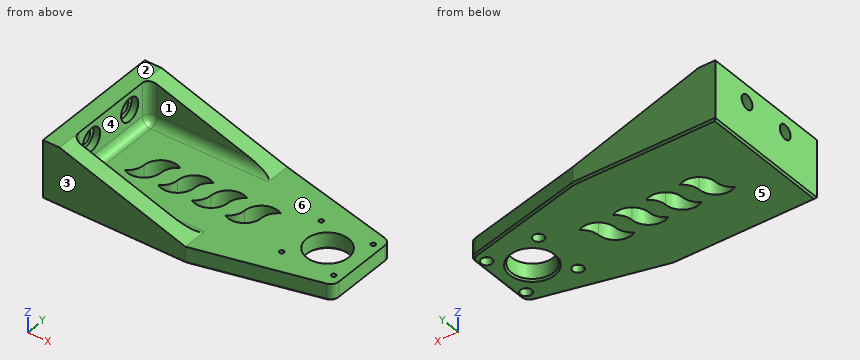
```python
from build123d import *

# Parameters (mm, degrees)
SKETCH1_W           = 160
SKETCH1_H           = 80
BOSS_EXTRUDE1_DEPTH = 10
SKETCH2_R           = 1.325
SKETCH2_R_2         = 12.5
CUT_EXTRUDE1_DEPTH  = 3
CUT_EXTRUDE2_REACH  = 9
SKETCH4_R           = 1.325
SKETCH4_R_2         = 12.5
SKETCH7_W           = 10
SKETCH7_H           = 80
BOSS_EXTRUDE3_DEPTH = 25
BOSS_EXTRUDE4_DEPTH = 10
BOSS_EXTRUDE5_DEPTH = 10
CUT_EXTRUDE3_REACH  = 12
CUT_EXTRUDE4_DEPTH  = 10
FILLET1_R           = 5
SKETCH12_R          = 3.25
CUT_EXTRUDE5_DEPTH  = 4.5
CUT_EXTRUDE6_REACH  = 12
SKETCH13_R          = 4.25
SKETCH14_R          = 6.75
CUT_EXTRUDE7_DEPTH  = 4
FILLET2_R           = 5
CHAMFER2_SIZE       = 1


with BuildPart() as part:
    # Sketch1 → Boss-Extrude1 (new body)
    with BuildSketch(Plane.XY):
        Rectangle(SKETCH1_W, SKETCH1_H)
    extrude(amount=BOSS_EXTRUDE1_DEPTH)

    # Sketch2 → Cut-Extrude1 (cut)
    with BuildSketch(Plane.XY.offset(10)):
        with Locations((44, 15.5)):
            Circle(SKETCH2_R)
        with Locations((75, 15.5)):
            Circle(SKETCH2_R)
        with Locations((44, -15.5)):
            Circle(SKETCH2_R)
        with Locations((75, -15.5)):
            Circle(SKETCH2_R)
        with Locations((59.5, 0)):
            Circle(SKETCH2_R_2)
    extrude(amount=-CUT_EXTRUDE1_DEPTH, mode=Mode.SUBTRACT)

    # Sketch4 → Cut-Extrude2 (cut, up to next)
    with BuildSketch(Plane.XY.offset(7), mode=Mode.PRIVATE) as cut_extrude2_sk1:
        with Locations((75, -15.5)):
            Circle(SKETCH4_R)
    cut_extrude2_tool1 = extrude(cut_extrude2_sk1.sketch, amount=-CUT_EXTRUDE2_REACH, mode=Mode.PRIVATE) & part.part
    add(cut_extrude2_tool1.solids().sort_by_distance((75, -15.5, 7))[0], mode=Mode.SUBTRACT)
    # Sketch4 → Cut-Extrude2 (cut, up to next)
    with BuildSketch(Plane.XY.offset(7), mode=Mode.PRIVATE) as cut_extrude2_sk2:
        with Locations((44, -15.5)):
            Circle(SKETCH4_R)
    cut_extrude2_tool2 = extrude(cut_extrude2_sk2.sketch, amount=-CUT_EXTRUDE2_REACH, mode=Mode.PRIVATE) & part.part
    add(cut_extrude2_tool2.solids().sort_by_distance((44, -15.5, 7))[0], mode=Mode.SUBTRACT)
    # Sketch4 → Cut-Extrude2 (cut, up to next)
    with BuildSketch(Plane.XY.offset(7), mode=Mode.PRIVATE) as cut_extrude2_sk3:
        with Locations((75, 15.5)):
            Circle(SKETCH4_R)
    cut_extrude2_tool3 = extrude(cut_extrude2_sk3.sketch, amount=-CUT_EXTRUDE2_REACH, mode=Mode.PRIVATE) & part.part
    add(cut_extrude2_tool3.solids().sort_by_distance((75, 15.5, 7))[0], mode=Mode.SUBTRACT)
    # Sketch4 → Cut-Extrude2 (cut, up to next)
    with BuildSketch(Plane.XY.offset(7), mode=Mode.PRIVATE) as cut_extrude2_sk4:
        with Locations((44, 15.5)):
            Circle(SKETCH4_R)
    cut_extrude2_tool4 = extrude(cut_extrude2_sk4.sketch, amount=-CUT_EXTRUDE2_REACH, mode=Mode.PRIVATE) & part.part
    add(cut_extrude2_tool4.solids().sort_by_distance((44, 15.5, 7))[0], mode=Mode.SUBTRACT)
    # Sketch4 → Cut-Extrude2 (cut, up to next)
    with BuildSketch(Plane.XY.offset(7), mode=Mode.PRIVATE) as cut_extrude2_sk5:
        with Locations((59.5, 0)):
            Circle(SKETCH4_R_2)
    cut_extrude2_tool5 = extrude(cut_extrude2_sk5.sketch, amount=-CUT_EXTRUDE2_REACH, mode=Mode.PRIVATE) & part.part
    add(cut_extrude2_tool5.solids().sort_by_distance((59.5, 0, 7))[0], mode=Mode.SUBTRACT)

    # Sketch7 → Boss-Extrude3 (add)
    with BuildSketch(Plane.XY.offset(10)):
        with Locations((-75, 0)):
            Rectangle(SKETCH7_W, SKETCH7_H)
    extrude(amount=BOSS_EXTRUDE3_DEPTH)

    # Sketch8 → Boss-Extrude4 (add)
    with BuildSketch(Plane(origin=(0, 40, 0), x_dir=(1, 0, 0), z_dir=(0, 1, 0))):
        Polygon((-70, -35), (5, -10), (-70, -10), align=None)
    extrude(amount=-BOSS_EXTRUDE4_DEPTH)

    # Sketch9 → Boss-Extrude5 (add)
    with BuildSketch(Plane.XZ.offset(40)):
        Polygon((-70, 35), (-70, 10), (5, 10), align=None)
    extrude(amount=-BOSS_EXTRUDE5_DEPTH)

    # Sketch10 → Cut-Extrude3 (cut, up to next)
    with BuildSketch(Plane.XY.offset(10), mode=Mode.PRIVATE) as cut_extrude3_sk1:
        with BuildLine():
            ThreePointArc((5, -8.660254038), (15, -8.660254038), (20, 0))
            ThreePointArc((20, 0), (21.339745962, 5), (25, 8.660254038))
            ThreePointArc((25, 8.660254038), (15, 8.660254038), (10, 0))
            ThreePointArc((10, 0), (8.660254038, -5), (5, -8.660254038))
        make_face()
    cut_extrude3_tool1 = extrude(cut_extrude3_sk1.sketch, amount=-CUT_EXTRUDE3_REACH, mode=Mode.PRIVATE) & part.part
    add(cut_extrude3_tool1.solids().sort_by_distance((15, 0, 10))[0], mode=Mode.SUBTRACT)
    # Sketch10 → Cut-Extrude3 (cut, up to next)
    with BuildSketch(Plane.XY.offset(10), mode=Mode.PRIVATE) as cut_extrude3_sk2:
        with BuildLine():
            ThreePointArc((0, 0), (1.339745962, 5), (5, 8.660254038))
            ThreePointArc((5, 8.660254038), (-5, 8.660254038), (-10, 0))
            ThreePointArc((-10, 0), (-11.339745962, -5), (-15, -8.660254038))
            ThreePointArc((-15, -8.660254038), (-5, -8.660254038), (0, 0))
        make_face()
    cut_extrude3_tool2 = extrude(cut_extrude3_sk2.sketch, amount=-CUT_EXTRUDE3_REACH, mode=Mode.PRIVATE) & part.part
    add(cut_extrude3_tool2.solids().sort_by_distance((-5, 0, 10))[0], mode=Mode.SUBTRACT)
    # Sketch10 → Cut-Extrude3 (cut, up to next)
    with BuildSketch(Plane.XY.offset(10), mode=Mode.PRIVATE) as cut_extrude3_sk3:
        with BuildLine():
            ThreePointArc((-20, 0), (-18.660254038, 5), (-15, 8.660254038))
            ThreePointArc((-15, 8.660254038), (-25, 8.660254038), (-30, 0))
            ThreePointArc((-30, 0), (-31.339745962, -5), (-35, -8.660254038))
            ThreePointArc((-35, -8.660254038), (-25, -8.660254038), (-20, 0))
        make_face()
    cut_extrude3_tool3 = extrude(cut_extrude3_sk3.sketch, amount=-CUT_EXTRUDE3_REACH, mode=Mode.PRIVATE) & part.part
    add(cut_extrude3_tool3.solids().sort_by_distance((-25, 0, 10))[0], mode=Mode.SUBTRACT)
    # Sketch10 → Cut-Extrude3 (cut, up to next)
    with BuildSketch(Plane.XY.offset(10), mode=Mode.PRIVATE) as cut_extrude3_sk4:
        with BuildLine():
            ThreePointArc((-40, 0), (-38.660254038, 5), (-35, 8.660254038))
            ThreePointArc((-35, 8.660254038), (-45, 8.660254038), (-50, 0))
            ThreePointArc((-50, 0), (-51.339745962, -5), (-55, -8.660254038))
            ThreePointArc((-55, -8.660254038), (-45, -8.660254038), (-40, 0))
        make_face()
    cut_extrude3_tool4 = extrude(cut_extrude3_sk4.sketch, amount=-CUT_EXTRUDE3_REACH, mode=Mode.PRIVATE) & part.part
    add(cut_extrude3_tool4.solids().sort_by_distance((-45, 0, 10))[0], mode=Mode.SUBTRACT)

    # Sketch11 → Cut-Extrude4 (cut)
    with BuildSketch(Plane.XY.offset(10)):
        Polygon((80, 22), (5, 40), (80, 40), align=None)
        Polygon((80, -40), (80, -22), (5, -40), align=None)
    extrude(amount=-CUT_EXTRUDE4_DEPTH, mode=Mode.SUBTRACT)

    # Fillet1
    fillet1_edges = [part.edges().sort_by_distance(p)[0] for p in [
        (-70, 30, 22.5),
        (-32.5, 30, 10),
        (-70, 0, 10),
        (-32.5, -30, 10),
        (-70, -30, 22.5),
    ]]
    fillet(fillet1_edges, radius=FILLET1_R)

    # Sketch12 → Cut-Extrude5 (cut)
    with BuildSketch(Plane(origin=(0, 0, 0), x_dir=(-1, 0, 0), z_dir=(0, 0, -1))):
        with Locations((-75, 15.5)):
            Circle(SKETCH12_R)
        with Locations((-44, 15.5)):
            Circle(SKETCH12_R)
        with Locations((-44, -15.5)):
            Circle(SKETCH12_R)
        with Locations((-75, -15.5)):
            Circle(SKETCH12_R)
    extrude(amount=-CUT_EXTRUDE5_DEPTH, mode=Mode.SUBTRACT)

    # Sketch13 → Cut-Extrude6 (cut, up to next)
    with BuildSketch(Plane(origin=(-70, 0, 0), x_dir=(0, 0, -1), z_dir=(1, 0, 0)), mode=Mode.PRIVATE) as cut_extrude6_sk1:
        with Locations((-25, 15)):
            Circle(SKETCH13_R)
    cut_extrude6_tool1 = extrude(cut_extrude6_sk1.sketch, amount=-CUT_EXTRUDE6_REACH, mode=Mode.PRIVATE) & part.part
    add(cut_extrude6_tool1.solids().sort_by_distance((-70, 15, 25))[0], mode=Mode.SUBTRACT)
    # Sketch13 → Cut-Extrude6 (cut, up to next)
    with BuildSketch(Plane(origin=(-70, 0, 0), x_dir=(0, 0, -1), z_dir=(1, 0, 0)), mode=Mode.PRIVATE) as cut_extrude6_sk2:
        with Locations((-25, -15)):
            Circle(SKETCH13_R)
    cut_extrude6_tool2 = extrude(cut_extrude6_sk2.sketch, amount=-CUT_EXTRUDE6_REACH, mode=Mode.PRIVATE) & part.part
    add(cut_extrude6_tool2.solids().sort_by_distance((-70, -15, 25))[0], mode=Mode.SUBTRACT)

    # Sketch14 → Cut-Extrude7 (cut)
    with BuildSketch(Plane(origin=(-70, 0, 0), x_dir=(0, 0, -1), z_dir=(1, 0, 0))):
        with Locations((-25, 15)):
            Circle(SKETCH14_R)
        with Locations((-25, -15)):
            Circle(SKETCH14_R)
    extrude(amount=-CUT_EXTRUDE7_DEPTH, mode=Mode.SUBTRACT)

    # Fillet2
    fillet2_edges = [part.edges().sort_by_distance(p)[0] for p in [
        (80, 22, 5),
        (80, -22, 5),
    ]]
    fillet(fillet2_edges, radius=FILLET2_R)

    # Chamfer2
    chamfer2_edges = [part.edges().sort_by_distance(p)[0] for p in [
        (-37.5, 40, 0),
        (40.583432381, 31.459976229, 0),
        (40.583432381, -31.459976229, 0),
        (80, 0, 0),
        (78.926469394, 21.153631895, 0),
        (78.926469394, -21.153631895, 0),
        (47, 0, 0),
        (-37.5, -40, 0),
        (-80, 0, 0),
    ]]
    chamfer(chamfer2_edges, length=CHAMFER2_SIZE)


solid = part.part
```
CAD build for the part. Positions are in the model's coordinates, mm. Face numbers are marked on the shaded views. A direction names the side the tool comes from. Round coordinates to 2 decimals unless told otherwise and drop trailing zeros. Write each loop counter-clockwise with the first axis right and the second up, starting at its lowest first coordinate (ties: lowest second). Pieces come first, ordered by that corner, then holes. Notation, with made-up numbers: M 26.25,67.25 L 67.25,67.25 A26 cw 67.25,99.25 Z; hole C 54,23.5 d3. An arc over 180 degrees is marked long. One line per question, with ' | ' between items.
1. Cut at B-B on z = 6. Count the separate pieces of the cut face and the enclosed holes in it, and give its area (3 significant figures).
Working result:
separate pieces: 1 | enclosed holes: 9 | area: 10,200 mm2
2. Cut at C-C on x = 59.5. Write the cut outline in (y, z), and give its area (3 significant figures).
Working result:
outline: M -26.92,1 L -25.89,0 L -13.5,0 L -12.5,1 L -12.5,10 L -26.92,10 Z; M 12.5,1 L 13.5,0 L 25.89,0 L 26.92,1 L 26.92,10 L 12.5,10 Z | area: 286 mm2
3. Which spindle directions (+Z, -Z, +X, -X, +Y, -Y) get a long thin tool onto all of the face, cutting with end or side? Do the marked faces 1 and 2. Say none if no direction does.
Working result:
face 1: +Z, +X | face 2: +Z, +X, -X, +Y, -Y
4. Mould opens along Y. For the marked faces 3, 4, 5 and 6 say: pulls with the +Y half, pulls with the -Y half, needs draft (parallel to the pull), parting line crosses it, or undercut.
Working result:
face 3: pulls with the -Y half | face 4: undercut | face 5: needs draft | face 6: undercut
5. Cut at A-A on z = 25. Write the cut outline in (x, y), and give its area (3 significant figures).
Working result:
outline: M -80,-40 L -40,-40 L -40,-30 L -65,-30 A5 cw -70,-25 L -70,-21.75 L -74,-21.75 L -74,-19.25 L -80,-19.25 Z; M -80,-10.75 L -74,-10.75 L -74,-8.25 L -70,-8.25 L -70,8.25 L -74,8.25 L -74,10.75 L -80,10.75 Z; M -80,19.25 L -74,19.25 L -74,21.75 L -70,21.75 L -70,25 A5 cw -65,30 L -40,30 L -40,40 L -80,40 Z | area: 1,200 mm2
6. Pin check, flat tips, straight feed: pin 1 Ø16 at (y, z) = (2, 20) entering from +X; pin 2 Ø3 at (x, y) = (76, 16) entering from -Z; pin 3 Ø24 at (x, y) = (-17, -14.5) entering from +Z. Stop position of each tip, or through.
Working result:
pin 1: x = -69 | pin 2: z = 4.5 | pin 3: z = 10.23
7. Probe L1, parallel to Y at x = -72, z = 25; L2, parallel to Y at x = 44, z = 8.5 (3 decimals); L3, parallel to Y at x = -35, z = 15. List the from-to ranges inside material, lowest first. Write a range as from..to.
Working result:
L1: -40..-21.75, -8.25..8.25, 21.75..40 | L2: -30.64..-16.825, -14.175..14.175, 16.825..30.64 | L3: -40..-30, 30..40
